Study the drawing (mm; zero at the part's minimum x, y, z) and answer. A direction names the side the tool comes from. Give positions to 0.01 mm unless a question says otherwise; leave off trailing zeros. Order: outer loops, then holes, each group sorted by start corner. A loop starts at its lowest first (then second) coordinate and runs counter-clockwise, first axis right, second up. Notation, with made-up numbers: (76.5, -14.5) -> (124.5, -14.5) arc R22 cw to (124.5, 6.5) -> close; hole circle Ø11 at (-6, 40.5). An arc over 180 degrees is marked (long way). Answer as CSV lines item,"result". Start each with the question number.
1. Flat-ended cylindrical pins translate along their axes: pin 1 (1 mm diameter, centred on x = 5.5, y = 10.5, fed in from +Z); pin 2 (6 mm diameter, centred on x = 3.5, y = 3, fed in from +Z); pin 3 (1.1 mm diameter, centred on x = 17.5, z = 10, fed in from -Y). Find the tip coordinate at first contact, or state that the pin passes through.
2. A cutting plane is placed at C-C (y = 10). Give the vertices of the cut face in (x, z).
3. For a pull along X with two mould halves and no side action, classify the marked faces 1, 2, 3 and 4 as released by +X, released by -X, zero draft, split by the parting line, or undercut.
4. A cutting plane is placed at D-D (z = 6.5). Give the vertices of the cut face in (x, y), then the cut area to 3 significant figures.
5. Find the intervals of material crossed by L1, parallel to Y at x = 10, z = 5; L2, parallel to X at y = 7, z = 10; L3, parallel to Z at x = 13.25, y = 2.5, in increasing order.
6. For the marked faces 5, 6 and 7, determine the directions among +Z, -Z, +X, -X, +Y, -Y from which every point of the face is accessible in a straight line to the end or side of a thin tool.
7. A cutting plane is placed at A-A (x = 10). Give the vertices of the cut face in (y, z), then the cut area to 3 significant figures.
8. A cutting plane is placed at B-B (z = 8.5). Give the vertices of the cut face in (x, y).
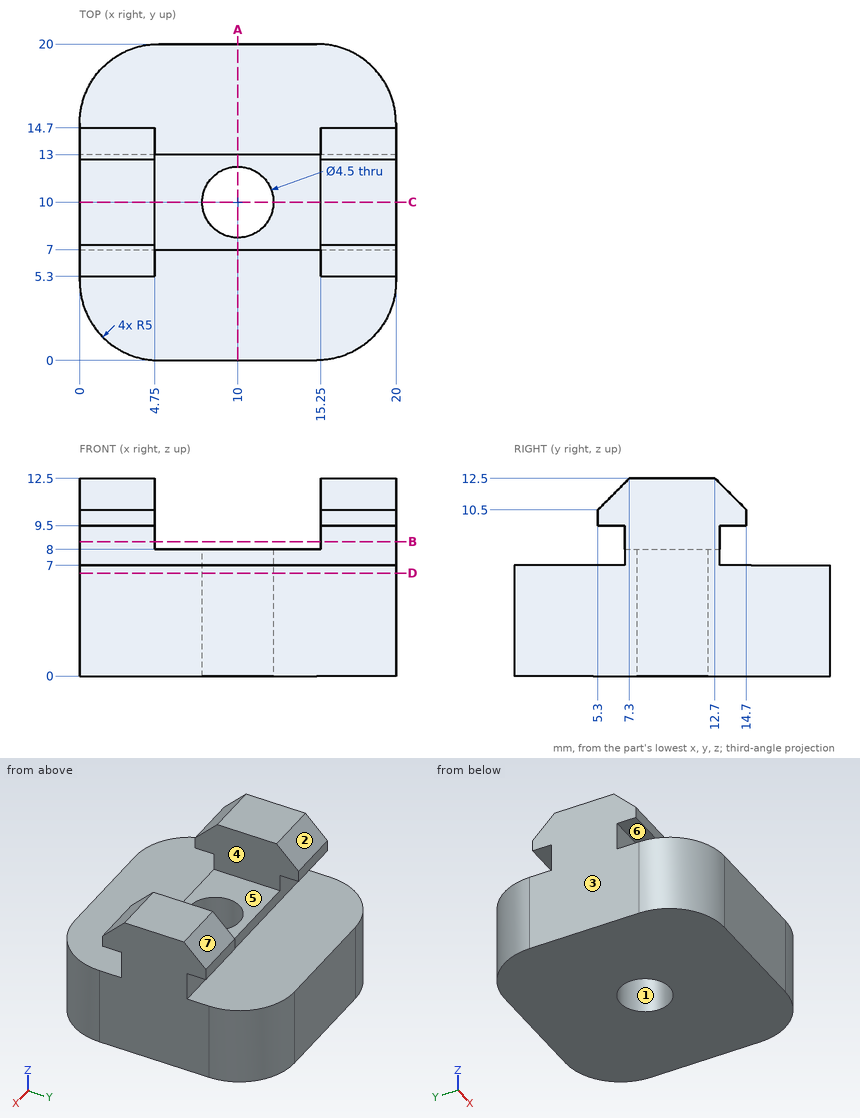
Answer sheet:
1,pin 1,"stops at z = 8"
1,pin 2,"stops at z = 11.2"
1,pin 3,"stops at y = 5.3"
2,outline,"(0, 0) -> (7.75, 0) -> (7.75, 8) -> (4.75, 8) -> (4.75, 12.5) -> (0, 12.5) -> close; (12.25, 0) -> (20, 0) -> (20, 12.5) -> (15.25, 12.5) -> (15.25, 8) -> (12.25, 8) -> close"
3,face 1,"undercut"
3,face 2,"zero draft"
3,face 3,"released by -X"
3,face 4,"undercut"
4,outline,"(0, 5) arc R5 ccw to (5, 0) -> (15, 0) arc R5 ccw to (20, 5) -> (20, 15) arc R5 ccw to (15, 20) -> (5, 20) arc R5 ccw to (0, 15) -> close; hole circle Ø4.5 at (10, 10)"
4,area,"363 mm^2"
5,L1,"y = 0 to 7.75, 12.25 to 20"
5,L2,"x = 0 to 4.75, 15.25 to 20"
5,L3,"z = 0 to 7"
6,face 5,"+Z, +Y, -Y"
6,face 6,"+X, -X, -Y"
6,face 7,"+Z, +X, -X, +Y"
7,outline,"(0, 0) -> (7.75, 0) -> (7.75, 8) -> (7, 8) -> (7, 7) -> (0, 7) -> close; (12.25, 0) -> (20, 0) -> (20, 7) -> (13, 7) -> (13, 8) -> (12.25, 8) -> close"
7,area,"110 mm^2"
8,outline,"(0, 7) -> (4.75, 7) -> (4.75, 13) -> (0, 13) -> close; (15.25, 7) -> (20, 7) -> (20, 13) -> (15.25, 13) -> close"
